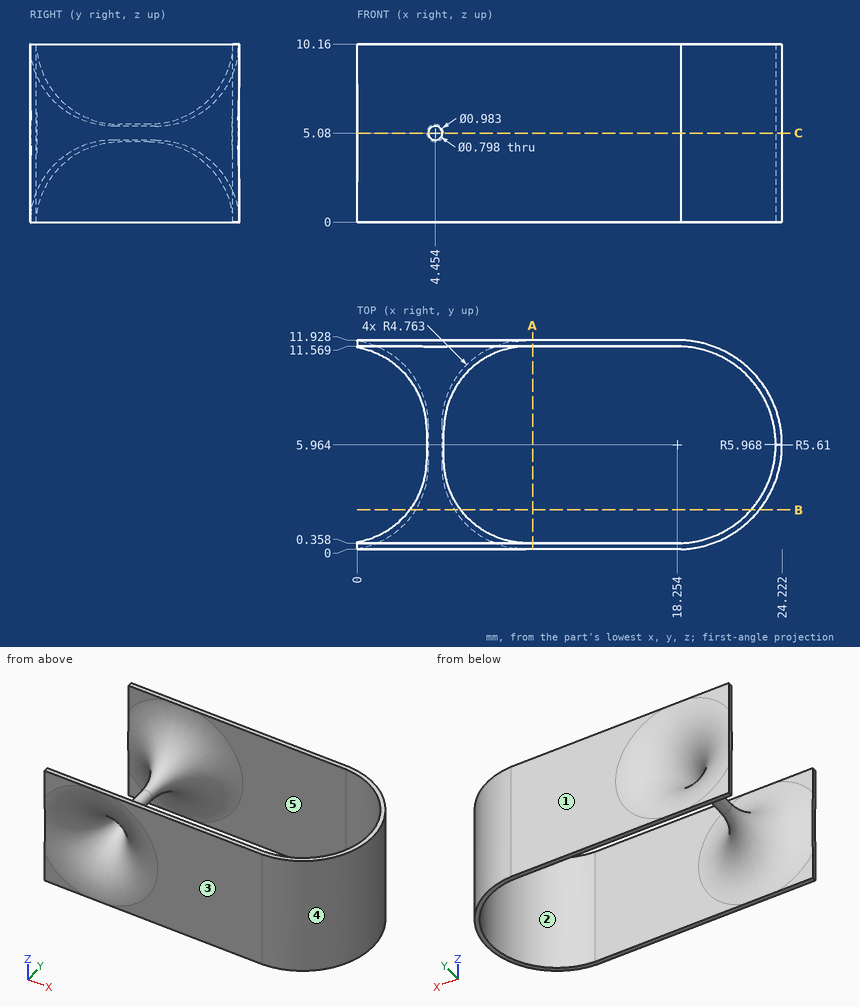
Here's the drawing with two shaded views (mm, measured from the low corner). I have some questions. A direction names the side the tool comes from. Round coordinates to 2 decimals unless told otherwise and drop trailing zeros. Write each loop counter-clockwise with the first axis right and the second up, starting at its lowest first coordinate (ties: lowest second). Pieces come first, ordered by that corner, then holes.
(1) If I drill on probe 1 along Y at (x, z) = (10, 9.5); probe 2 along Y at (x, z) = (20, 7.75) (1 decimal); probe 3 along X at (y, z) = (4, 2.5), over which ranges is the centre line in solid material (lowest first)?
Findings below:
probe 1: y = 0 to 0.36, 11.57 to 11.93
probe 2: y = 0.3 to 0.6, 11.3 to 11.7
probe 3: x = 23.51 to 23.89
(2) Suppose I cut it at A-A on x = 10. Write out the boundary of the cut face in (y, z).
Findings below:
outline: (0, 0) - (0.36, 0) - (0.36, 10.16) - (0, 10.16) - close; (11.57, 0) - (11.93, 0) - (11.93, 10.16) - (11.57, 10.16) - close
(3) Which directions (+Z, -Z, +X, -X, +Y, -Y) give clear straight access to the entire face, cutting with the end or side of a thin tool? Please do the marked faces 1 and 2.
Findings below:
face 1: +Z, -Z, +X, -X, +Y
face 2: +Z, -Z
(4) Suppose I cut it at B-B on y = 2.25. Write out the boundary of the cut face in (x, z) (1 decimal).
Findings below:
outline: circle Ø2.9 at (4.5, 5.1); (22.5, 0) - (22.9, 0) - (22.9, 10.2) - (22.5, 10.2) - close; hole circle Ø2.2 at (4.5, 5.1)
(5) Suppose I cut it at C-C on z = 5.08. State how many separate pieces and enclosed holes the cut face has.
Findings below:
separate pieces: 2
enclosed holes: 1
(6) Thinking about a two-plate mould opening in Y: for the marked faces 3, 4 and 5, which applies, +Y half, -Y half, draft (parallel to the pull), parting line (faces both ways), or undercut?
Findings below:
face 3: -Y half
face 4: parting line
face 5: undercut
